Geometry: final body of the model. Coordinates: model frame, mm. Round coordinates to 2 decimals unless told otherwise and drop trailing zeros. Loops run counter-clockwise (first coordinate to the right, second up) from the corner with the lowest first, then second, coordinate; pieces in that order, holes last. Notation, with made-up numbers: (82, -33.75) -> (93, -33.75) arc R31 ccw to (93, 5.25) -> close; hole circle Ø6 at (89, 39.5). An arc over 180 degrees is marked (long way). Answer in a Markdown table with one row per item.
Solid Edge part; units mm, degrees
sketch "Sketch1" plane through (0, 0, 0) normal (0, 0, 1) x (1, 0, 0)
  line L0 (-2, 0) -> (-2, 12)
  line L1 (-2, 12) -> (-1.1265, 14.4)
  line L2 (-1.1265, 14.4) -> (1.1265, 14.4)
  line L3 (1.1265, 14.4) -> (2, 12)
  line L4 (2, 12) -> (2, 0)
  line L5 (2, 0) -> (-2, 0)
revolve "RevolvedProtrusion1" add sketch "Sketch1" angle 360 about axis through (2, 0, 0) along (-1, 0, 0)
sketch "Sketch2" plane through (0, 0, 0) normal (1, 0, 0) x (0, 1, 0)
  line L0 (24, 24) -> (-24, 24)
  line L1 (-24, 24) -> (-24, -24)
  line L2 (-24, -24) -> (24, -24)
  line L3 (24, -24) -> (24, 24)
  line L4 (-6.9282, 12) -> (-13.8564, 0)
  line L5 (-13.8564, 0) -> (-6.9282, -12)
  line L6 (-6.9282, -12) -> (6.9282, -12)
  line L7 (6.9282, -12) -> (13.8564, 0)
  line L8 (13.8564, 0) -> (6.9282, 12)
  line L9 (6.9282, 12) -> (-6.9282, 12)
extrude "Extrusionsausschnitt_1" cut sketch "Sketch2" against normal blind 4 and the other way blind 4
sketch "Sketch3" plane through (0, 0, 0) normal (0, 0, 1) x (1, 0, 0)
  line L0 (-2, 0) -> (-2, 9)
  line L1 (-2, 9) -> (-1.4585, 8.4585)
  line L2 (-1.4585, 8.4585) -> (1.4585, 8.4585)
  line L3 (1.4585, 8.4585) -> (2, 9)
  line L4 (2, 9) -> (2, 0)
  line L5 (2, 0) -> (-2, 0)
revolve "RevolvedCutout1" cut sketch "Sketch3" angle 360 about axis through (2, 0, 0) along (-1, 0, 0)
properties part number "Nut M18 x 1"
Item 1: Cut plane A-A (x = 0.65). Output: boundary loops of the cut face in (y, z).
Answer:
| item | result |
|---|---|
| outline | (-13.86, 0) -> (-6.93, -12) -> (6.93, -12) -> (13.86, 0) -> (6.93, 12) -> (-6.93, 12) -> close; hole circle Ø16.92 at (0, 0) |
Item 2: Draft query along Z for faces 1 (the face through (0.02, -6.23, 5.72)), 2 (the face through (0.03, 10.44, 5.92)), 3 (the face through (-1.86, 12.38, -0.03)). Return one class per face: pulls with the +Z half, pulls with the -Z half, needs draft (parallel to the pull), parting line crosses it, or undercut.
Answer:
| item | result |
|---|---|
| face 1 | undercut |
| face 2 | pulls with the +Z half |
| face 3 | parting line crosses it |
Item 3: Pin query (flat end, axial travel): pin 1 Ø1.5 at (x, z) = (0, 0.5) entering from +Y. Return the tip coordinate at first contact, or that it passes through.
Answer:
| item | result |
|---|---|
| pin 1 | stops at y = 13.86 |
Item 4: Line query: probe 1 along Z at (x, y) = (0.5, 0); probe 2 along Z at (x, y) = (-0.4, 0.5); probe 3 along Y at (x, z) = (0.75, -3). Output: solid intervals per line, ascending. Write a range as [from, to].
Answer:
| item | result |
|---|---|
| probe 1 | z = [-12, -8.46], [8.46, 12] |
| probe 2 | z = [-12, -8.44], [8.44, 12] |
| probe 3 | y = [-12.12, -7.91], [7.91, 12.12] |
